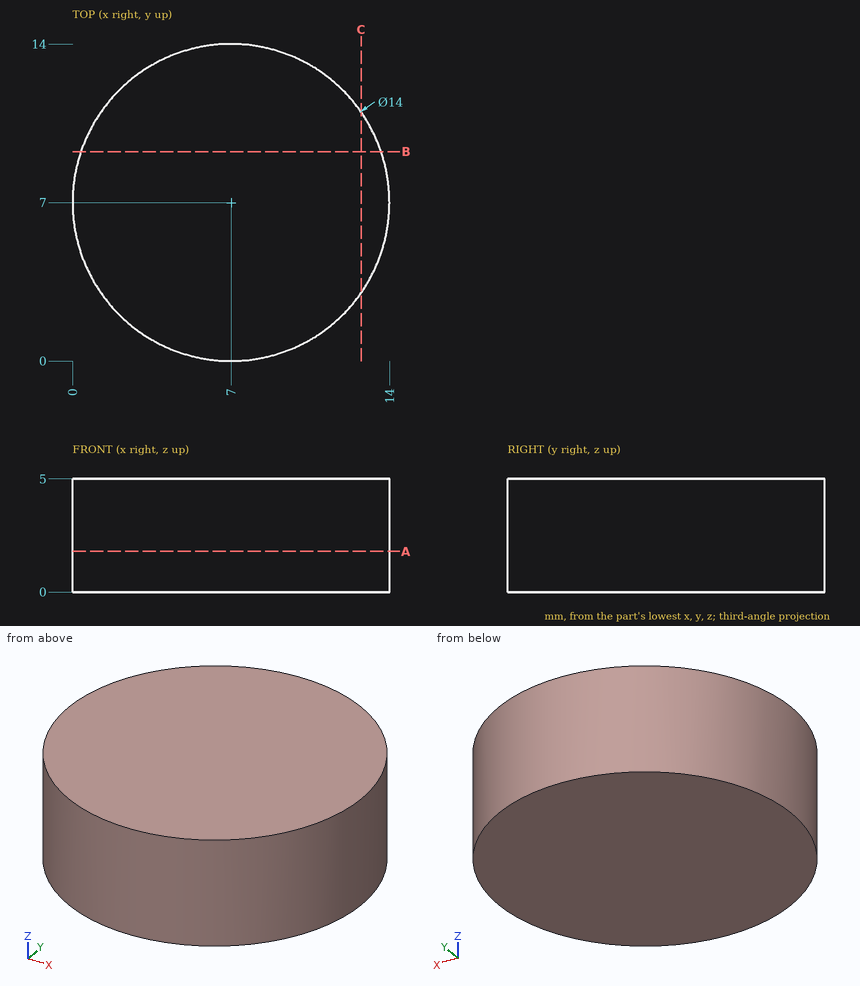
Job drawing, mm, ordinate dimensions from the low corner. One solid piece. Give positions to 0.01 mm unless a question says otherwise; leave off trailing zeros. Order: outer loops, then holes, each group sorted by start corner. A loop starts at its lowest first (then second) coordinate and runs counter-clockwise, first axis right, second up. Notation, with made-up numbers: M 57.5,35.5 L 79.5,35.5 A13 cw 79.5,44.5 Z; hole C 75,83 d2. An arc over 180 degrees is marked long. Put each result on its own line as item: value. Start each with the question number.
(1) Band-saw the part on C-C on x = 12.75. Give the cut face in (y, z), then the cut area to 3 significant figures.
(2) Band-saw the part on B-B on y = 9.25. Give the cut face in (x, z).
(3) Band-saw the part on A-A on z = 1.8. Give the cut face in (x, y), then the cut area to 3 significant figures.
(4) Pin check, flat tips, straight feed: pin 1 Ø4 at (x, y) = (11.5, 10) entering from -Z; pin 2 Ø2 at (y, z) = (12, 3.5) entering from -X. Stop position of each tip, or through.
(5) Drill centre lines: L1, parallel to X at y = 6.75, z = 0.3; L2, parallel to Y at x = 13, z = 3.1; L3, parallel to Y at x = 9.75, z = 2.8. Where is each one in solid material? Low to high. Write a range as [from, to].
Results below:
1. outline: M 3.01,0 L 10.99,0 L 10.99,5 L 3.01,5 Z
1. area: 39.9 mm2
2. outline: M 0.37,0 L 13.63,0 L 13.63,5 L 0.37,5 Z
3. outline: C 7,7 d14
3. area: 154 mm2
4. pin 1: stops at z = 0
4. pin 2: stops at x = 1.26
5. L1: x = [0, 14]
5. L2: y = [3.39, 10.61]
5. L3: y = [0.56, 13.44]
